```python
from build123d import *

# Parameters (mm, degrees)
SKETCH1_W           = 85
SKETCH1_H           = 75.1
SKETCH1_R           = 1.7
BOSS_EXTRUDE1_DEPTH = 3.175


with BuildPart() as part:
    # Sketch1 → Boss-Extrude1 (new body)
    with BuildSketch(Plane(origin=(0, 0, 0), x_dir=(0, 0, -1), z_dir=(1, 0, 0))):
        with Locations((42.5, 37.55)):
            Rectangle(SKETCH1_W, SKETCH1_H)
        with Locations((9, 65.05)):
            Circle(SKETCH1_R, mode=Mode.SUBTRACT)
        with Locations(Location((9, 10.05, 0), (0, 0, 180))):
            Circle(SKETCH1_R, mode=Mode.SUBTRACT)
        with Locations((76, 10.05)):
            Circle(SKETCH1_R, mode=Mode.SUBTRACT)
        with Locations(Location((76, 65.05, 0), (0, 0, 180))):
            Circle(SKETCH1_R, mode=Mode.SUBTRACT)
    extrude(amount=BOSS_EXTRUDE1_DEPTH)


solid = part.part
```
Here's how the part is built. I have some questions about the finished solid (model axes, mm). Coordinates: 2 decimals unless noted, no trailing zeros. Write each loop counter-clockwise with the first axis right and the second up, starting at its lowest first coordinate (ties: lowest second). Pieces come first, ordered by that corner, then holes. Notation, with made-up numbers: M 75.25,41.25 L 119.25,41.25 A15 cw 119.25,57.25 Z; hole C 68,-30.75 d7. An arc over 180 degrees is marked long. Answer as CSV lines item,"result". Start each with the question number.
Q1. I need wall thicknesses on probe 1 along Y at (x, z) = (1.35, -9); probe 2 along Z at (x, y) = (1.2, 65.05); probe 3 along Z at (x, y) = (1.9, 8.5). Which ranges of each line are inside material? Lowest first, please. Write a range as [from, to].
Q2. If we mould it in two halves opening along Z, with no side actions, what happens to faces 1 (the flat face through (2, 37, -85)), 2 (the flat face through (2, 0, -42)), 3 (the cylindrical face through (1.57, 63.39, -8.63)), 4 (the cylindrical face through (1.57, 66.08, -77.35))? For each: pulls with the +Z half, pulls with the -Z half, needs draft (parallel to the pull), parting line crosses it, or undercut.
Q3. Suppose I cut it at B-B, the plane y = 65.05. List the corners of the cut face in (x, z) for me (3 decimals), then the cut area to 3 significant figures.
Q4. Suppose I cut it at A-A, the plane z = -76. List the corners of the cut face in (x, y) for me (3 decimals).
Q5. Will these pins go through, and if not, where does the flat tip stop? pin 1 Ø4 at (y, z) = (65.05, -76) entering from -X; pin 2 Ø2.5 at (y, z) = (10.05, -9) entering from -X.
Entries:
1,probe 1,"y = [0, 8.35], [11.75, 63.35], [66.75, 75.1]"
1,probe 2,"z = [-85, -77.7], [-74.3, -10.7], [-7.3, 0]"
1,probe 3,"z = [-85, -76.7], [-75.3, -9.7], [-8.3, 0]"
2,face 1,"pulls with the -Z half"
2,face 2,"needs draft"
2,face 3,"undercut"
2,face 4,"undercut"
3,outline,"M 0,-85 L 3.175,-85 L 3.175,-77.7 L 0,-77.7 Z; M 0,-74.3 L 3.175,-74.3 L 3.175,-10.7 L 0,-10.7 Z; M 0,-7.3 L 3.175,-7.3 L 3.175,0 L 0,0 Z"
3,area,"248 mm²"
4,outline,"M 0,0 L 3.175,0 L 3.175,8.35 L 0,8.35 Z; M 0,11.75 L 3.175,11.75 L 3.175,63.35 L 0,63.35 Z; M 0,66.75 L 3.175,66.75 L 3.175,75.1 L 0,75.1 Z"
5,pin 1,"stops at x = 0"
5,pin 2,"passes through"
